```python
from build123d import *

# Parameters (mm, degrees)
SKETCH1_R           = 8.1
BOSS_EXTRUDE1_DEPTH = 100
SKETCH2_R           = 14.4
CUT_EXTRUDE1_DEPTH  = 80
CUT_EXTRUDE2_START  = -80
CUT_EXTRUDE2_DEPTH  = 80
SKETCH4_R           = 14.4
CUT_EXTRUDE3_DEPTH  = 15
SKETCH8_W           = 32.8
SKETCH8_H           = 80
CUT_EXTRUDE4_DEPTH  = 106.913171985
CUT_EXTRUDE5_START  = -2
SKETCH9_R           = 4.1
CUT_EXTRUDE5_DEPTH  = 3.1


with BuildPart() as part:
    # Sketch1 → Boss-Extrude1 (new body)
    with BuildSketch(Plane(origin=(0, 0, 0), x_dir=(1, 0, 0), z_dir=(0, 1, 0))):
        with BuildLine():
            Line((-16.4, 0), (-16.4, 21.4))
            Line((-16.4, 21.4), (16.4, 21.4))
            Line((16.4, 21.4), (16.4, 0))
            ThreePointArc((16.4, 0), (0, -16.4), (-16.4, 0))
        make_face()
        with Locations(Location((0, 0, 0), (0, 0, 270))):
            Circle(SKETCH1_R, mode=Mode.SUBTRACT)
    extrude(amount=BOSS_EXTRUDE1_DEPTH)

    # Sketch2 → Cut-Extrude1 (cut)
    with BuildSketch(Plane(origin=(0, 100, 0), x_dir=(1, 0, 0), z_dir=(0, 1, 0))):
        with Locations(Location((0, 0, 0), (0, 0, 270))):
            Circle(SKETCH2_R)
    extrude(amount=-CUT_EXTRUDE1_DEPTH, mode=Mode.SUBTRACT)

    # Sketch3 → Cut-Extrude2 (cut)
    with BuildSketch(Plane(origin=(0, 100, 0), x_dir=(1, 0, 0), z_dir=(0, 1, 0)).offset(CUT_EXTRUDE2_START)):
        with BuildLine():
            Line((-16.4, 0), (-16.4, 14.4))
            Line((-16.4, 14.4), (16.4, 14.4))
            Line((16.4, 14.4), (16.4, 0))
            ThreePointArc((16.4, 0), (0, -16.4), (-16.4, 0))
        make_face()
    extrude(amount=CUT_EXTRUDE2_DEPTH, mode=Mode.SUBTRACT)

    # Sketch4 → Cut-Extrude3 (cut)
    with BuildSketch(Plane(origin=(0, 20, 0), x_dir=(1, 0, 0), z_dir=(0, 1, 0))):
        with Locations(Location((0, 0, 0), (0, 0, 270))):
            Circle(SKETCH4_R)
    extrude(amount=-CUT_EXTRUDE3_DEPTH, mode=Mode.SUBTRACT)

    # Sketch8 → Cut-Extrude4 (cut, through all)
    with BuildSketch(Plane.XY.offset(-14.4)):
        with Locations((0, 60)):
            Rectangle(SKETCH8_W, SKETCH8_H)
    extrude(amount=-CUT_EXTRUDE4_DEPTH, mode=Mode.SUBTRACT)

    # Sketch9 → Cut-Extrude5 (cut)
    with BuildSketch(Plane(origin=(0, 20, 0), x_dir=(1, 0, 0), z_dir=(0, 1, 0)).offset(CUT_EXTRUDE5_START)):
        with Locations(Location((-11.366921431, 16.176228268, 0), (0, 0, 270))):
            Circle(SKETCH9_R)
    cut_extrude5 = extrude(amount=-CUT_EXTRUDE5_DEPTH, mode=Mode.SUBTRACT)

    # Mirror1: Cut-Extrude5 across plane
    add(cut_extrude5.mirror(Plane(origin=(0, 0, 0), x_dir=(0, 0, 1), z_dir=(1, 0, 0))), mode=Mode.SUBTRACT)


solid = part.part
```
Work out the finished part from the listing and answer in its coordinate system (mm). A direction names the side the tool comes from. Give positions to 0.01 mm unless a question says otherwise; leave off trailing zeros. Write each loop counter-clockwise with the first axis right and the second up, starting at its lowest first coordinate (ties: lowest second). Pieces come first, ordered by that corner, then holes. Notation, with made-up numbers: (75, 31) - (107, 31) arc R34 cw to (107, 67) - close; hole circle Ø4 at (65.5, -35). An arc over 180 degrees is marked (long way). Use one line per item in the form item = value.
1. A cutting plane is placed at D-D (x = -12.5). Write down the section's boundary in (y, z).
Filled in:
outline = (0, -21.4) - (20, -21.4) - (20, -7.15) - (5, -7.15) - (5, 7.15) - (20, 7.15) - (20, 10.62) - (0, 10.62) - close; hole (14.9, -20.12) - (18, -20.12) - (18, -12.24) - (14.9, -12.24) - close
2. A cutting plane is placed at A-A (x = 0). Write down the section's boundary in (y, z).
Filled in:
outline = (0, -21.4) - (20, -21.4) - (20, -14.4) - (5, -14.4) - (5, -8.1) - (0, -8.1) - close; (0, 8.1) - (5, 8.1) - (5, 14.4) - (20, 14.4) - (20, 16.4) - (0, 16.4) - close
3. Determine the mould class of faces 4 (the face through (-11, 14.9, -16)), 5 (the face through (0, 10, -21.4)), 6 (the face through (0.361, 9.86, 16.396)) for opening direction X: released by +X, released by -X, zero draft, split by the parting line, or undercut.
Filled in:
face_4 = undercut
face_5 = zero draft
face_6 = split by the parting line
4. A cutting plane is placed at C-C (y = 17). Write down the section's boundary in (x, z).
Filled in:
outline = (-16.4, -21.4) - (16.4, -21.4) - (16.4, 0) arc R16.4 ccw to (-16.4, 0) - close; hole circle Ø8.2 at (-11.37, -16.18); hole circle Ø28.8 at (0, 0); hole circle Ø8.2 at (11.37, -16.18)
5. Each of these flat-tipped pins is pushed along its axis until it touches: pin 1 Ø2 at (x, y) = (2, 8.5) entering from +Z; pin 2 Ø5 at (y, z) = (9.5, 7) entering from -X; pin 3 Ø4 at (y, z) = (16.5, 12.5) entering from -X; pin 4 Ø13 at (x, z) = (0, 0) entering from -Y (3 decimals). Where does it stop, or does it pass through?
Filled in:
pin_1 = 16.37
pin_2 = -15.77
pin_3 = -12.6
pin_4 = through
6. For faces 1 (the face through (-7.3, 16.5, -16.7)), 2 (the face through (16.4, 10, -11)), 3 (the face through (-6, 5, 6)), determine the directions among +Z, -Z, +X, -X, +Y, -Y from which every point of the face is accessible in a straight line to the end or side of a thin tool.
Filled in:
face_1 = none
face_2 = +Z, -Z, +X, +Y, -Y
face_3 = +Y
7. Consider L1, parallel to Y at x = -9, z = -0.5; L2, parallel to Z at x = -0.5, y = 14; L3, parallel to X at y = 17.5, z = 2.5. Determine where each line is inside the solid, lowest interval first.
Filled in:
L1 = 0 to 5
L2 = -21.4 to -14.39, 14.39 to 16.39
L3 = -16.21 to -14.18, 14.18 to 16.21
8. A cutting plane is placed at B-B (z = 3). Write down the section's boundary in (x, y).
Filled in:
outline = (-16.12, 0) - (-7.52, 0) - (-7.52, 5) - (-14.08, 5) - (-14.08, 20) - (-16.12, 20) - close; (7.52, 0) - (16.12, 0) - (16.12, 20) - (14.08, 20) - (14.08, 5) - (7.52, 5) - close
